Read the model definition and answer for the solid it produces. Units are mm, in the model's axes. Face numbers are marked on the shaded views. Round coordinates to 2 decimals unless told otherwise and drop trailing zeros. Write each loop counter-clockwise with the first axis right and the second up, starting at its lowest first coordinate (ties: lowest second). Pieces come first, ordered by that corner, then holes. Notation, with made-up numbers: (13.25, 81.25) - (62.25, 81.25) arc R4 cw to (62.25, 88.25) - close; hole circle Ø10 at (27, 12). An arc over 180 degrees is marked (long way). Answer as CSV lines item,"result". Start each with the question number.
1) Find section A-A on z = 0. Determine the outline of the cut face in (x, y), then the cut area to 3 significant figures.
2) For a pull along X with two mould halves and no side action, classify the marked faces 1, 2 and 3 as +X half, -X half, draft (parallel to the pull), parting line (faces both ways), or undercut.
3) Find section B-B on x = 0. Determine the outline of the cut face in (y, z), then the cut area to 3 significant figures.
4) Find section C-C on y = -53.5. Determine the outline of the cut face in (x, z).
5) Consider line 1 along Z through (x, y) = (0, -27); line 2 along X through (y, z) = (-44.5, 13); line 3 along Z through (x, y) = (-8.5, -18.5). Determine where each line is inside the solid, lowest interval first.
6) Each of these flat-tipped pins is pushed along its axis until it touches: pin 1 (3 mm diameter, centred on x = 7, y = -32, fed in from +Z); pin 2 (2 mm diameter, centred on x = 5, y = -42.5, fed in from -Z); pin 3 (10 mm diameter, centred on y = -48, z = 13.5, fed in from -X); pin 4 (1.5 mm diameter, centred on x = -11, z = 13.5, fed in from +Y). Where does it stop, or does it pass through?
from build123d import *

# Parameters (mm, degrees)
F0_R     = 22.5
F1_DEPTH = 64
F2_R     = 4
F3_DEPTH = 64
F4_R     = 5


with BuildPart() as f1:
    # F0 (on Front) → F1 (new body)
    with BuildSketch(Plane.XZ):
        Circle(F0_R)
    extrude(amount=F1_DEPTH)

    # F2 (on face) → F3 (cut)
    with BuildSketch(Plane(origin=(0, 0, 0), x_dir=(-1, 0, 0), z_dir=(0, 1, 0))):
        Circle(F2_R)
    extrude(amount=-F3_DEPTH, mode=Mode.SUBTRACT)

    # F4
    f4_edges = [f1.edges().sort_by_distance(p)[0] for p in [
        (-22.5, -64, 0),
        (-22.5, 0, 0),
    ]]
    fillet(f4_edges, radius=F4_R)


solid = f1.part
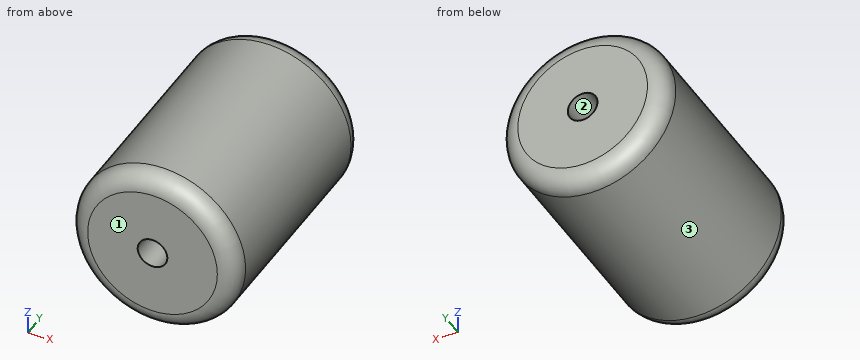
Check values:
1,outline,"(-22.5, -59) arc R5 ccw to (-17.5, -64) - (-4, -64) - (-4, 0) - (-17.5, 0) arc R5 ccw to (-22.5, -5) - close; (4, -64) - (17.5, -64) arc R5 ccw to (22.5, -59) - (22.5, -5) arc R5 ccw to (17.5, 0) - (4, 0) - close"
1,area,"2,350 mm^2"
2,face 1,"draft"
2,face 2,"undercut"
2,face 3,"parting line"
3,outline,"(-64, -17.5) arc R5 ccw to (-59, -22.5) - (-5, -22.5) arc R5 ccw to (0, -17.5) - (0, -4) - (-64, -4) - close; (-64, 4) - (0, 4) - (0, 17.5) arc R5 ccw to (-5, 22.5) - (-59, 22.5) arc R5 ccw to (-64, 17.5) - close"
3,area,"2,350 mm^2"
4,outline,"circle Ø45 at (0, 0); hole circle Ø8 at (0, 0)"
5,line 1,"z = -22.5 to -4, 4 to 22.5"
5,line 2,"x = -18.36 to 18.36"
5,line 3,"z = -20.83 to 20.83"
6,pin 1,"stops at z = 21.82"
6,pin 2,"stops at z = -22.14"
6,pin 3,"stops at x = -20.83"
6,pin 4,"stops at y = 0"
